Work out the finished part from the listing and answer in its coordinate system (mm). A direction names the side the tool comes from. Coordinates: 2 decimals unless noted, no trailing zeros. Write each loop counter-clockwise with the first axis right and the second up, starting at its lowest first coordinate (ties: lowest second). Pieces come first, ordered by that corner, then holes. Notation, with made-up numbers: (34.25, 86) - (57.25, 86) arc R26 cw to (57.25, 117) - close; hole circle Ø9 at (-30, 25). An arc over 180 degrees is marked (long way). Use a Markdown table: item, result. Add a question column.
(1) Given pin 1 Ø1.5 at (y, z) = (-0.5, 15.5) entering from +X; pin 2 Ø1.5 at (y, z) = (5, 20) entering from -X; pin 3 Ø3.5 at (x, y) = (-28.6, 7.9) entering from +Z; pin 4 Ø3 at (x, y) = (14.4, 5) entering from -Z, each flat-ended and moving along its own axis, determine where each tip first touches the part or whether it passes through.
(2) Find the intervals of material crossed by line 1 (Y direction, x = -35, z = 29); line 2 (X direction, y = 7.9, z = 1.15); line 3 (X direction, y = 7.9, z = 1.65), in increasing order. Write a range as from..to.
(3) The part is cut by section A-A, the plane z = 19. Give the vertices of the cut face in (x, y), then the cut area to 3 significant figures.
(4) The part is cut by section B-B, the plane x = -1. Give the vertices of the cut face in (y, z), then the cut area to 3 significant figures.
(5) A tool of negligible diameter and unlimited length cuts with its end or side. For faces 1 (the face through (-29, 8, 2)), 2 (the face through (9.4, -9.33, 14.94)), 3 (the face through (-30.03, 9.3, 33.53)), 4 (the face through (-30.03, 9.3, 14.94)), 5 (the face through (-30.03, -9.3, 14.94)), from which of +Z, -Z, +X, -X, +Y, -Y can it reach the whole face along a straight path? Write none if from no direction.
(6) The part is cut by section C-C, the plane y = 0. Give the vertices of the cut face in (x, z), then the cut area to 3 significant figures.
from build123d import *

# Parameters (mm, degrees)
SKETCH007_R      = 6
EXTRUDE007_DEPTH = 1.3
SKETCH008_R      = 5
EXTRUDE008_DEPTH = 0.9
SKETCH004_W      = 5
SKETCH004_H      = 2.5
EXTRUDE004_DEPTH = 3
SKETCH003_R      = 2
EXTRUDE003_DEPTH = 3
SKETCH002_W      = 54.6
SKETCH002_H      = 3
EXTRUDE002_DEPTH = 19.8
SKETCH001_R      = 1.5
EXTRUDE001_DEPTH = 2
SKETCH_W         = 40.6
SKETCH_H         = 19.8
EXTRUDE_DEPTH    = 36
FILLET_R         = 2
CHAMFER_SIZE     = 1.5
FILLET001_R      = 0.5
FILLET002_R      = 2
SKETCH005_R      = 9
EXTRUDE005_DEPTH = 2
SKETCH006_W      = 23.9
SKETCH006_H      = 15
EXTRUDE006_DEPTH = 2


with BuildPart() as extrude007:
    # Sketch007 (on Face81 of Fusion002) → Extrude007 (new body)
    with BuildSketch(Plane.XY.offset(38)):
        Circle(SKETCH007_R)
    extrude(amount=EXTRUDE007_DEPTH)


with BuildPart() as extrude008:
    # Sketch008 (on Face3 of Extrude007) → Extrude008 (new body)
    with BuildSketch(Plane.XY.offset(39.3)):
        Circle(SKETCH008_R)
    extrude(amount=EXTRUDE008_DEPTH)


with BuildPart() as extrude004:
    # Sketch004 (on Face13 of Cut001) → Extrude004 (new body)
    with BuildSketch(Plane.XY.offset(31)):
        with Locations((-37.5, 5)):
            Rectangle(SKETCH004_W, SKETCH004_H)
        with Locations((16.9, 5)):
            Rectangle(SKETCH004_W, SKETCH004_H)
        with Locations((16.9, -5)):
            Rectangle(SKETCH004_W, SKETCH004_H)
        with Locations((-37.5, -5)):
            Rectangle(SKETCH004_W, SKETCH004_H)
    extrude(amount=-EXTRUDE004_DEPTH)


with BuildPart() as extrude003:
    # Sketch003 (on Face11 of Fillet002) → Extrude003 (new body)
    with BuildSketch(Plane.XY.offset(31)):
        with Locations((-35, 5)):
            Circle(SKETCH003_R)
        with Locations((-35, -5)):
            Circle(SKETCH003_R)
        with Locations((14.4, 5)):
            Circle(SKETCH003_R)
        with Locations((14.4, -5)):
            Circle(SKETCH003_R)
    extrude(amount=-EXTRUDE003_DEPTH)


with BuildPart() as extrude002:
    # Sketch002 (on Face6 of Fillet001) → Extrude002 (new body)
    with BuildSketch(Plane.XZ.offset(9.9)):
        with Locations((-10.3, 29.5)):
            Rectangle(SKETCH002_W, SKETCH002_H)
    extrude(amount=-EXTRUDE002_DEPTH)


with BuildPart() as extrude001:
    # Sketch001 (on Face8 of Chamfer) → Extrude001 (new body)
    with BuildSketch(Plane(origin=(0, 0, 0), x_dir=(1, 0, 0), z_dir=(0, 0, -1))):
        with Locations((-28.6, 7.9)):
            Circle(SKETCH001_R)
        with Locations((8, 7.9)):
            Circle(SKETCH001_R)
        with Locations((-28.6, -7.9)):
            Circle(SKETCH001_R)
        with Locations((8, -7.9)):
            Circle(SKETCH001_R)
    extrude(amount=-EXTRUDE001_DEPTH)


with BuildPart() as cut002:
    # Sketch → Extrude (new body)
    with BuildSketch(Plane.XY):
        with Locations((-10.3, 0)):
            Rectangle(SKETCH_W, SKETCH_H)
    extrude(amount=EXTRUDE_DEPTH)

    # Fillet
    fillet_edges = [cut002.edges().sort_by_distance(p)[0] for p in [
        (-30.6, -9.9, 18),
        (10, -9.9, 18),
        (10, 9.9, 18),
        (-30.6, 9.9, 18),
    ]]
    fillet(fillet_edges, radius=FILLET_R)

    # Chamfer
    chamfer_edges = [cut002.edges().sort_by_distance(p)[0] for p in [
        (-10.3, -9.9, 0),
        (-30.014214, -9.314214, 0),
        (9.414214, -9.314214, 0),
        (-30.6, 0, 0),
        (10, 0, 0),
        (-30.014214, 9.314214, 0),
        (9.414214, 9.314214, 0),
        (-10.3, 9.9, 0),
    ]]
    chamfer(chamfer_edges, length=CHAMFER_SIZE)

    # Cut: cut Extrude001
    add(extrude001.part, mode=Mode.SUBTRACT)

    # Fillet001
    fillet001_edges = [cut002.edges().sort_by_distance(p)[0] for p in [
        (-27.733975, -6.675255, 0),
        (-27.733975, 6.675255, 0),
        (6.93934, 6.83934, 0),
        (6.93934, -6.83934, 0),
    ]]
    fillet(fillet001_edges, radius=FILLET001_R)

    # Fusion: union Extrude002
    add(extrude002.part)

    # Fillet002
    fillet002_edges = [cut002.edges().sort_by_distance(p)[0] for p in [
        (-37.6, -9.9, 29.5),
        (-37.6, 9.9, 29.5),
        (17, -9.9, 29.5),
        (17, 9.9, 29.5),
    ]]
    fillet(fillet002_edges, radius=FILLET002_R)

    # Cut001: cut Extrude003
    add(extrude003.part, mode=Mode.SUBTRACT)

    # Cut002: cut Extrude004
    add(extrude004.part, mode=Mode.SUBTRACT)


with BuildPart() as extrude005:
    # Sketch005 (on Face48 of Cut002) → Extrude005 (new body)
    with BuildSketch(Plane.XY.offset(36)):
        Circle(SKETCH005_R)
    extrude(amount=EXTRUDE005_DEPTH)


with BuildPart() as fusion003:
    # Sketch006 (on Face48 of Cut002) → Extrude006 (new body)
    with BuildSketch(Plane.XY.offset(36)):
        with Locations((-11.95, 0)):
            Rectangle(SKETCH006_W, SKETCH006_H)
    extrude(amount=EXTRUDE006_DEPTH)

    # Fusion001: union Extrude005
    add(extrude005.part)

    # Fusion002: union Cut002
    add(cut002.part)

    # Fusion003: union Extrude007, Extrude008
    add(extrude007.part)
    add(extrude008.part)


solid = fusion003.part
Model answer:
| question | item | result |
|---|---|---|
| 1 | pin 1 | x = 10 |
| 1 | pin 2 | x = -30.6 |
| 1 | pin 3 | z = 36 |
| 1 | pin 4 | through |
| 2 | line 1 | -9.9..-7, -3..3, 7..9.9 |
| 2 | line 2 | -30.25..-30.1, -27.1..6.5, 9.5..9.65 |
| 2 | line 3 | -30.6..-30.1, -27.1..6.5, 9.5..10 |
| 3 | outline | (-30.6, -7.9) arc R2 ccw to (-28.6, -9.9) - (8, -9.9) arc R2 ccw to (10, -7.9) - (10, 7.9) arc R2 ccw to (8, 9.9) - (-28.6, 9.9) arc R2 ccw to (-30.6, 7.9) - close |
| 3 | area | 800 mm^2 |
| 4 | outline | (-9.9, 1.5) - (-8.4, 0) - (8.4, 0) - (9.9, 1.5) - (9.9, 36) - (8.94, 36) - (8.94, 38) - (5.92, 38) - (5.92, 39.3) - (4.9, 39.3) - (4.9, 40.2) - (-4.9, 40.2) - (-4.9, 39.3) - (-5.92, 39.3) - (-5.92, 38) - (-8.94, 38) - (-8.94, 36) - (-9.9, 36) - close |
| 4 | area | 771 mm^2 |
| 5 | face 1 | -Z |
| 5 | face 2 | -Z, +X, -Y |
| 5 | face 3 | +Z, -X, +Y |
| 5 | face 4 | -Z, -X, +Y |
| 5 | face 5 | -Z, -X, -Y |
| 6 | outline | (-37.6, 28) - (-30.6, 28) - (-30.6, 1.5) - (-29.1, 0) - (8.5, 0) - (10, 1.5) - (10, 28) - (17, 28) - (17, 31) - (10, 31) - (10, 36) - (9, 36) - (9, 38) - (6, 38) - (6, 39.3) - (5, 39.3) - (5, 40.2) - (-5, 40.2) - (-5, 39.3) - (-6, 39.3) - (-6, 38) - (-23.9, 38) - (-23.9, 36) - (-30.6, 36) - (-30.6, 31) - (-37.6, 31) - close |
| 6 | area | 1,590 mm^2 |
